Geometry check sheet. Reference: the model listing, model coordinates, mm. A direction names the side the tool comes from. Round coordinates to 2 decimals unless told otherwise and drop trailing zeros. Loops run counter-clockwise (first coordinate to the right, second up) from the corner with the lowest first, then second, coordinate; pieces in that order, holes last. Notation, with made-up numbers: M 59.5,45.25 L 86.5,45.25 A20 ccw 86.5,51.25 Z; hole C 89,18.25 d1. An arc over 180 degrees is marked long. Answer in a Markdown table with one row per item. Add a question column.
```python
from build123d import *

# Parameters (mm, degrees)
SKETCH1_W                   = 61.88
SKETCH1_H                   = 39.878
BOSS_EXTRUDE1_DEPTH         = 3
F_32_0_116_DIAMETER_HOLE1_D = 2.9464
FILLET1_R                   = 2.54
SKETCH6_W                   = 12.7
SKETCH6_H                   = 3
CUT_EXTRUDE1_DEPTH          = 3
SKETCH7_W                   = 19.05
SKETCH7_H                   = 3.81
CUT_EXTRUDE2_DEPTH          = 74.67760368
FILLET2_R                   = 1.27
CUT_EXTRUDE4_DEPTH          = 3


with BuildPart() as part:
    # Sketch1 → Boss-Extrude1 (new body)
    with BuildSketch(Plane.XY):
        with Locations((30.94, 19.939)):
            Rectangle(SKETCH1_W, SKETCH1_H)
    extrude(amount=BOSS_EXTRUDE1_DEPTH)

    # #32 (0.116) Diameter Hole1 (through all)
    with Locations(Plane.XY.offset(3)):
        with Locations((30.94, 6.373999952), (59.11, 32.7152), (2.77, 32.7152)):
            Hole(F_32_0_116_DIAMETER_HOLE1_D / 2)

    # Fillet1
    fillet1_edges = [part.edges().sort_by_distance(p)[0] for p in [
        (61.88, 0, 1.5),
        (0, 0, 1.5),
    ]]
    fillet(fillet1_edges, radius=FILLET1_R)

    # Sketch6 → Cut-Extrude1 (cut)
    with BuildSketch(Plane(origin=(0, 0, 0), x_dir=(-1, 0, 0), z_dir=(0, 0, -1))):
        with Locations((-30.9428, 38.378)):
            Rectangle(SKETCH6_W, SKETCH6_H)
    extrude(amount=-CUT_EXTRUDE1_DEPTH, mode=Mode.SUBTRACT)

    # Sketch7 → Cut-Extrude2 (cut, through all)
    with BuildSketch(Plane(origin=(0, 0, 0), x_dir=(-1, 0, 0), z_dir=(0, 0, -1))):
        with Locations((-30.9428, 1.905)):
            Rectangle(SKETCH7_W, SKETCH7_H)
    extrude(amount=-CUT_EXTRUDE2_DEPTH, mode=Mode.SUBTRACT)

    # Fillet2
    fillet2_edges = [part.edges().sort_by_distance(p)[0] for p in [
        (40.4678, 0, 1.5),
        (40.4678, 3.81, 1.5),
        (21.4178, 3.81, 1.5),
        (21.4178, 0, 1.5),
    ]]
    fillet(fillet2_edges, radius=FILLET2_R)

    # Sketch10 → Cut-Extrude4 (cut)
    with BuildSketch(Plane(origin=(0, 0, 0), x_dir=(-1, 0, 0), z_dir=(0, 0, -1))):
        with BuildLine():
            ThreePointArc((-10.60427198, 22.930843482), (-18.715027328, 17.096117028), (-13.486198066, 25.610089641))
            ThreePointArc((-13.486198066, 25.610089641), (-14.439521527, 21.695056792), (-10.60427198, 22.930843482))
        make_face()
        with BuildLine():
            ThreePointArc((-41.99867198, 22.930843482), (-45.833921527, 21.695056792), (-44.880598066, 25.610089641))
            ThreePointArc((-44.880598066, 25.610089641), (-50.109427328, 17.096117028), (-41.99867198, 22.930843482))
        make_face()
    extrude(amount=-CUT_EXTRUDE4_DEPTH, mode=Mode.SUBTRACT)


solid = part.part
```
1) Cross-section at C-C, the plane x = 45.5. Record the boundary of the cut face in (y, z).
2) Draft check along Y on faces 4 (the cylindrical face through (40.106, 3.428, 1.521)), 5 (the cylindrical face through (32.41, 6.44, 1.48)), 6 (the flat face through (31, 36.878, 1)). Enter one of: +Y half, -Y half, draft (parallel to the pull), parting line (faces both ways), or undercut.
3) Cross-section at B-B, the plane z = 1. Record the boundary of the cut face in (x, y), plus the area to 3 significant figures.
4) Cross-section at A-A, the plane x = 30.94. Record the boundary of the cut face in (y, z), plus the area to 3 significant figures.
5) Go/stop test with flat-tipped pins: pin 1 (1 mm diameter, centred on x = 36.5, y = 8.5, fed in from -Z); pin 2 (1.8 mm diameter, centred on x = 30.94, y = 6.374, fed in from -Z); pin 3 (0.9 mm diameter, centred on x = 30.5, z = 2, fed in from +Y); pin 4 (1.4 mm diameter, centred on y = 1.5, z = 2, fed in from +X). Record where each tip stops, or that it passes through.
6) Set-up check for faces 1 (the flat face through (24.593, 38, 1)), 2 (the flat face through (31, 3.81, 1)), 3 (the cylindrical face through (0.724, 0.764, 1.521)): record each of +Z, -Z, +X, -X, +Y, -Y from which the full face is reachable in a straight line by a thin tool's end or side.
7) Thickness scan on L1, parallel to Y at x = 31, z = 2.25; L2, parallel to X at y = 25, z = 1.55; L3, parallel to Y at x = 14, z = 1.15. Record the ranges inside material, lowest first. Write a range as [from, to].
Worked answers:
| question | item | result |
|---|---|---|
| 1 | outline | M 0,0 L 15.86,0 L 15.86,3 L 0,3 Z; M 21.44,0 L 25.33,0 L 25.33,3 L 21.44,3 Z; M 25.79,0 L 39.88,0 L 39.88,3 L 25.79,3 Z |
| 2 | face 4 | -Y half |
| 2 | face 5 | undercut |
| 2 | face 6 | +Y half |
| 3 | outline | M 0,2.54 A2.54 ccw 2.54,0 L 20.15,0 A1.27 ccw 21.42,1.27 L 21.42,2.54 A1.27 cw 22.69,3.81 L 39.2,3.81 A1.27 cw 40.47,2.54 L 40.47,1.27 A1.27 ccw 41.74,0 L 59.34,0 A2.54 ccw 61.88,2.54 L 61.88,39.88 L 37.29,39.88 L 37.29,36.88 L 24.59,36.88 L 24.59,39.88 L 0,39.88 Z; hole C 2.77,32.72 d2.95; hole M 10.6,22.93 A5.1 ccw long 13.49,25.61 A2.31 cw long Z; hole C 30.94,6.37 d2.95; hole M 42,22.93 A5.1 ccw long 44.88,25.61 A2.31 cw long Z; hole C 59.11,32.72 d2.95 |
| 3 | area | 2,200 mm2 |
| 4 | outline | M 3.81,0 L 4.9,0 L 4.9,3 L 3.81,3 Z; M 7.85,0 L 36.88,0 L 36.88,3 L 7.85,3 Z |
| 4 | area | 90.4 mm2 |
| 5 | pin 1 | stops at z = 0 |
| 5 | pin 2 | passes through |
| 5 | pin 3 | stops at y = 36.88 |
| 5 | pin 4 | stops at x = 61.86 |
| 6 | face 1 | +Z, -Z, +Y |
| 6 | face 2 | +Z, -Z, -Y |
| 6 | face 3 | +Z, -Z, -X, -Y |
| 7 | L1 | y = [3.81, 4.9], [7.85, 36.88] |
| 7 | L2 | x = [0, 14.52], [18.17, 45.91], [49.57, 61.88] |
| 7 | L3 | y = [0, 15.89], [21.37, 25.4], [25.77, 39.88] |
